Geometry check sheet. Reference: the model listing, model coordinates, mm. Face numbers are marked on the shaded views. A direction names the side the tool comes from. Coordinates: 2 decimals unless noted, no trailing zeros. Write each loop counter-clockwise with the first axis right and the second up, starting at its lowest first coordinate (ties: lowest second). Pieces come first, ordered by that corner, then holes. Notation, with made-up numbers: M 6.5,-40 L 61.5,-40 A8 ccw 61.5,-31 Z; hole C -16.5,-10.5 d1. An arc over 180 degrees is marked long. Put each result on its own line as item: value. Start each with the question number.
1) Cross-section at B-B on x = 17. Record the cut outline in (y, z).
2) Scan lines: line 1 along Z through (x, y) = (21.75, -4.25); line 2 along X through (y, z) = (-1.75, -7); line 3 along Z through (x, y) = (26, 4.5). Record each from-to range of solid material in increasing order.
3) Cross-section at C-C on y = 2. Record the cut outline in (x, z), plus the area to 3 significant figures.
4) Cross-section at A-A on x = 21. Record the cut outline in (y, z).
5) Gauge pin test, flat ends, axial feed: pin 1 (1 mm diameter, centred on x = 19, y = -2, fed in from -Z); pin 2 (3.5 mm diameter, centred on x = 18.08, y = 5.93, fed in from +Z). Record the tip position at first contact, or that the pin passes through.
6) Mould release check, pull along Z, two halves, no side actions. Record for the marked faces 1, 2 and 3: released by +Z, released by -Z, zero draft, split by the parting line, or undercut.
7) Set-up check for the marked faces 4 and 5: record each of +Z, -Z, +X, -X, +Y, -Y from which the full face is reachable in a straight line by a thin tool's end or side.
8) Cross-section at D-D on z = -7.5. Record the cut outline in (x, y), plus the area to 3 significant figures.
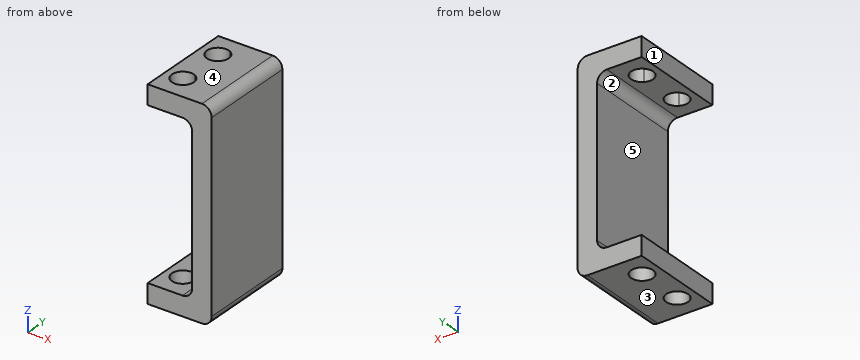
Autodesk Inventor part; units mm, degrees
ref_plane "YZ Plane" through (0, 0, 0) normal (1, 0, 0) x (0, 1, 0)
ref_plane "XZ Plane" through (0, 0, 0) normal (0, 1, 0) x (-1, 0, 0)
ref_plane "XY Plane" through (0, 0, 0) normal (0, 0, 1) x (1, 0, 0)
sketch "Эскиз1" plane through (0, 0, 0) normal (0, 0, 1) x (1, 0, 0)
  line L0 (21.232, 7.9335) -> (21.232, 9.4835)
  arc A0 (21.232, 9.4835) -> (19.732, 10.9835) centre (19.732, 9.4835) ccw
  line L1 (19.732, 10.9835) -> (-31.568, 10.9835)
  line L2 (-31.568, -9.0165) -> (19.732, -9.0165)
  arc A1 (19.732, -9.0165) -> (21.232, -7.5165) centre (19.732, -7.5165) ccw
  line L3 (21.232, -7.5165) -> (21.232, -5.9665)
  line L4 (21.232, -5.9665) -> (19.1128, -5.9665)
  arc A2 (19.1128, -1.9665) -> (19.1128, -5.9665) centre (18.082, -3.9665) ccw
  line L5 (19.1128, -1.9665) -> (21.232, -1.9665)
  line L6 (21.232, -1.9665) -> (21.232, 3.9335)
  line L7 (21.232, 3.9335) -> (19.1128, 3.9335)
  arc A3 (19.1128, 7.9335) -> (19.1128, 3.9335) centre (18.082, 5.9335) ccw
  line L8 (19.1128, 7.9335) -> (21.232, 7.9335)
  line L9 (-24.768, -8.9965) -> (13.532, -8.9965)
  line L10 (13.532, 10.9635) -> (-24.768, 10.9635)
  arc A4 (14.512, 9.9835) -> (13.532, 10.9635) centre (13.532, 9.9835) ccw
  line L11 (14.512, -8.0165) -> (14.512, 9.9835)
  arc A5 (13.532, -8.9965) -> (14.512, -8.0165) centre (13.532, -8.0165) ccw
  line L12 (14.512, 9.9835) -> (14.512, 13.5721)
  line L13 (21.652, -9.0165) -> (14.512, -9.0165)
  line L14 (14.512, -9.0165) -> (14.512, 10.9835)
  line L15 (14.512, 10.9835) -> (21.652, 10.9835)
  line L16 (21.652, 10.9835) -> (21.652, -9.0165)
  line L17 (21.652, -9.0165) -> (14.512, 10.9835) construction
  line L18 (14.512, -9.0165) -> (21.652, 10.9835) construction
  circle A6 centre (18.082, 5.9335) radius 2.25
  circle A7 centre (18.082, -3.9665) radius 2.25
  line L19 (21.652, 10.9835) -> (23.652, 10.9835)
  line L20 (23.652, 10.9835) -> (23.652, -9.0165)
  line L21 (23.652, -9.0165) -> (21.652, -9.0165)
  line L22 (21.652, -9.0165) -> (21.652, 10.9835)
  point P0 (0, 0)
  point P1 (-5.918, 0.9835)
  point P2 (18.082, 0.9835)
  point P3 (19.1128, -5.9665)
  point P4 (19.732, -9.0165)
  dimension "d2" = 2
extrude "Выдавливание1" add sketch "Эскиз1" along normal blind 4 contours L8 A3 L7 L6 L5 A2 L4 L3 A1 L2 L14 L11 L12 L1 A0 L0 | L0 A0 L15 L16 L13 A1 L3 L4 A7 L5 L6 L7 A6 L8 | L19 L20 L21 L16
sketch "Эскиз2" plane through (0, 0, 4) normal (0, 0, 1) x (1, 0, 0)
  line L0 (23.652, 10.9835) -> (14.512, 10.9835)
  line L1 (14.512, 10.9835) -> (14.512, -9.0165)
  line L2 (14.512, -9.0165) -> (23.652, -9.0165)
  line L3 (23.652, -9.0165) -> (23.652, 10.9835)
  circle A0 centre (18.082, -3.9665) radius 2.25
  circle A1 centre (18.082, 5.9335) radius 2.25
  line L4 (23.652, 10.9835) -> (27.652, 10.9835)
  line L5 (27.652, 10.9835) -> (27.652, -9.0165)
  line L6 (27.652, -9.0165) -> (23.652, -9.0165)
  line L7 (23.652, -9.0165) -> (23.652, 10.9835)
  point P0 (0, 0)
  dimension "d3" = 4
extrude "Выдавливание2" add sketch "Эскиз2" against normal blind 42 contours L4 L5 L6 L3
sketch "Эскиз3" plane through (0, 0, -38) normal (0, 0, -1) x (-1, 0, 0)
  line L0 (-23.652, 10.9835) -> (-14.512, 10.9835)
  line L1 (-23.652, -9.0165) -> (-23.652, 10.9835)
  line L2 (-14.512, -9.0165) -> (-23.652, -9.0165)
  line L3 (-14.512, 10.9835) -> (-14.512, -9.0165)
  circle A0 centre (-18.082, -3.9665) radius 2.25
  circle A1 centre (-18.082, 5.9335) radius 2.25
  point P0 (0, 0)
extrude "Выдавливание3" add sketch "Эскиз3" against normal blind 4
fillet "Сопряжение1" radius 2 4 edges at (23.652, 0.9835, 0) (23.652, 0.9835, -34) (27.652, 0.9835, -38) (27.652, 0.9835, 4)
properties part number "крепл сервы на пуляло"
Answer key:
1. outline: M -9.02,-38 L -5.94,-38 L -5.94,-34 L -9.02,-34 Z; M -9.02,0 L -5.94,0 L -5.94,4 L -9.02,4 Z; M -1.99,-38 L 3.96,-38 L 3.96,-34 L -1.99,-34 Z; M -1.99,0 L 3.96,0 L 3.96,4 L -1.99,4 Z; M 7.91,-38 L 10.98,-38 L 10.98,-34 L 7.91,-34 Z; M 7.91,0 L 10.98,0 L 10.98,4 L 7.91,4 Z
2. line 1: z = -38 to -34, 0 to 4
2. line 2: x = 23.65 to 27.65
2. line 3: z = -37.97 to 3.97
3. outline: M 14.51,-38 L 25.65,-38 A2 ccw 27.65,-36 L 27.65,2 A2 ccw 25.65,4 L 14.51,4 L 14.51,0 L 21.65,0 A2 cw 23.65,-2 L 23.65,-32 A2 cw 21.65,-34 L 14.51,-34 Z
3. area: 241 mm²
4. outline: M -9.02,-38 L 10.98,-38 L 10.98,-34 L -9.02,-34 Z; M -9.02,0 L 10.98,0 L 10.98,4 L -9.02,4 Z
5. pin 1: stops at z = -38
5. pin 2: passes through
6. face 1: zero draft
6. face 2: undercut
6. face 3: released by -Z
7. face 4: +Z, +X, -X, +Y, -Y
7. face 5: -X, +Y, -Y
8. outline: M 23.65,-9.02 L 27.65,-9.02 L 27.65,10.98 L 23.65,10.98 Z
8. area: 80.0 mm²
